Could you check a few things on this drawing? It's one solid part, dimensions in mm from its lowest x, y, z. Round coordinates to 2 decimals unless told otherwise and drop trailing zeros. Loops run counter-clockwise (first coordinate to the right, second up) from the corner with the lowest first, then second, coordinate; pieces in that order, holes last.
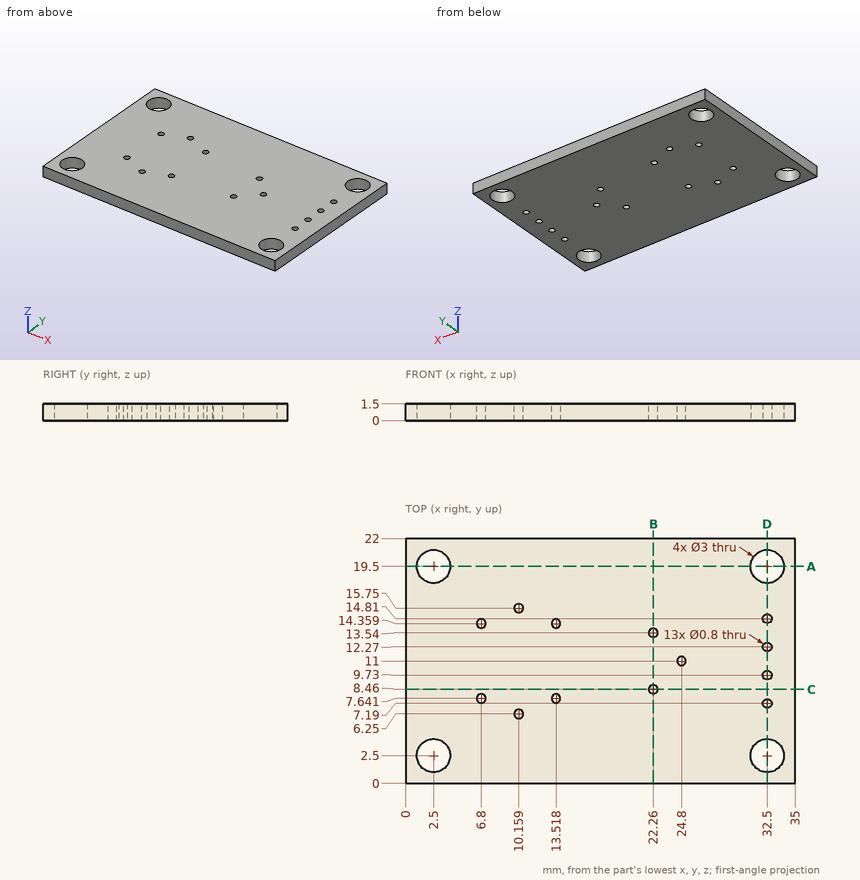
(1) Suppose I cut it at C-C (y = 8.46). Write out the boundary of the cut face in (x, z).
(2) If I drill on line 1 (Y direction, x = 6.8, z = 1); line 2 (Y direction, x = 22.26, z = 0.75); line 3 (X direction, y = 2.5, z = 1.1), over which ranges is the centre line in solid material (lowest first)?
(3) Suppose I cut it at B-B (x = 22.26). Write out the boundary of the cut face in (y, z).
(4) Suppose I cut it at D-D (x = 32.5). Write out the boundary of the cut face in (y, z).
(5) For pin 1 (3.5 mm diameter, centred on x = 2.5, y = 19.5, fed in from -Z); pin 2 (1.8 mm diameter, centred on x = 2.5, y = 2.5, fed in from -Z), each with a flat end and sliding along its axis, tell me the tip position at first contact or that it passes through.
(6) Suppose I cut it at A-A (y = 19.5). Write out the boundary of the cut face in (x, z).
Check result:
1. outline: (0, 0) - (21.86, 0) - (21.86, 1.5) - (0, 1.5) - close; (22.66, 0) - (35, 0) - (35, 1.5) - (22.66, 1.5) - close
2. line 1: y = 0 to 7.24, 8.04 to 13.96, 14.76 to 22
2. line 2: y = 0 to 8.06, 8.86 to 13.14, 13.94 to 22
2. line 3: x = 0 to 1, 4 to 31, 34 to 35
3. outline: (0, 0) - (8.06, 0) - (8.06, 1.5) - (0, 1.5) - close; (8.86, 0) - (13.14, 0) - (13.14, 1.5) - (8.86, 1.5) - close; (13.94, 0) - (22, 0) - (22, 1.5) - (13.94, 1.5) - close
4. outline: (0, 0) - (1, 0) - (1, 1.5) - (0, 1.5) - close; (4, 0) - (6.79, 0) - (6.79, 1.5) - (4, 1.5) - close; (7.59, 0) - (9.33, 0) - (9.33, 1.5) - (7.59, 1.5) - close; (10.13, 0) - (11.87, 0) - (11.87, 1.5) - (10.13, 1.5) - close; (12.67, 0) - (14.41, 0) - (14.41, 1.5) - (12.67, 1.5) - close; (15.21, 0) - (18, 0) - (18, 1.5) - (15.21, 1.5) - close; (21, 0) - (22, 0) - (22, 1.5) - (21, 1.5) - close
5. pin 1: stops at z = 0
5. pin 2: passes through
6. outline: (0, 0) - (1, 0) - (1, 1.5) - (0, 1.5) - close; (4, 0) - (31, 0) - (31, 1.5) - (4, 1.5) - close; (34, 0) - (35, 0) - (35, 1.5) - (34, 1.5) - close
